from build123d import *

# Parameters (mm, degrees)
BOSS_EXTRUDE1_DEPTH     = 30
SKETCH3_R               = 1.4
CUT_EXTRUDE1_DEPTH      = 5
MIRROR2_COPY_1_SKETCH_R = 1.4
MIRROR2_COPY_1_DEPTH    = 5


with BuildPart() as part:
    # Sketch2 → Boss-Extrude1 (new body)
    with BuildSketch(Plane(origin=(0, 0, 0), x_dir=(1, 0, 0), z_dir=(0, 1, 0))):
        with BuildLine():
            ThreePointArc((6.25, 13.635890143), (0, 15), (-6.25, 13.635890143))
            ThreePointArc((-6.25, 13.635890143), (-7.727178029, 9.658712115), (-3.75, 8.181534086))
            ThreePointArc((-3.75, 8.181534086), (0, 9), (3.75, 8.181534086))
            ThreePointArc((3.75, 8.181534086), (7.727178029, 9.658712115), (6.25, 13.635890143))
        make_face()
    extrude(amount=BOSS_EXTRUDE1_DEPTH)

    # Sketch3 → Cut-Extrude1 (cut)
    with BuildSketch(Plane(origin=(0, 30, 0), x_dir=(1, 0, 0), z_dir=(0, 1, 0))):
        with Locations(Location((5, 10.908712115, 0), (0, 0, 270))):
            Circle(SKETCH3_R)
    cut_extrude1 = extrude(amount=-CUT_EXTRUDE1_DEPTH, mode=Mode.SUBTRACT)

    # Mirror1: Cut-Extrude1 across plane
    add(cut_extrude1.mirror(Plane(origin=(0, 0, 0), x_dir=(0, 0, 1), z_dir=(1, 0, 0))), mode=Mode.SUBTRACT)

    # Mirror2: Cut-Extrude1 across plane
    add(cut_extrude1.mirror(Plane.ZX.offset(15)), mode=Mode.SUBTRACT)

    # Mirror2 copy 1 sketch → Mirror2 copy 1 (cut)
    with BuildSketch(Plane(origin=(0, 0, 0), x_dir=(-1, 0, 0), z_dir=(0, -1, 0))):
        with Locations(Location((5, 10.908712115, 0), (0, 0, 270))):
            Circle(MIRROR2_COPY_1_SKETCH_R)
    extrude(amount=-MIRROR2_COPY_1_DEPTH, mode=Mode.SUBTRACT)


solid = part.part
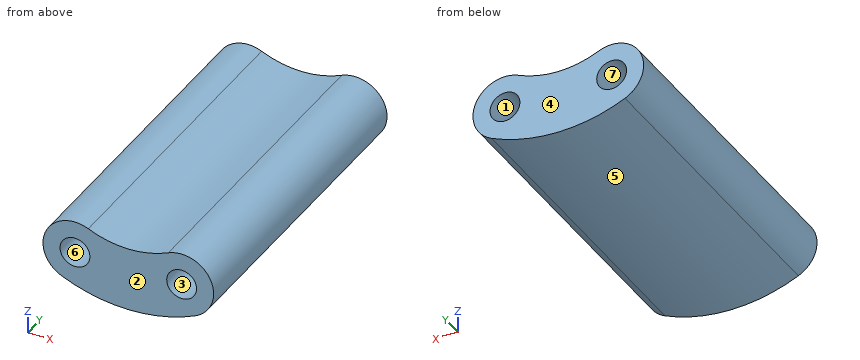
Design review of the part built by this model. Coordinates are the model's own, in mm. Face numbers are marked on the shaded views. A direction names the side the tool comes from. Give positions to 0.01 mm unless a question says otherwise; leave off trailing zeros. Loops run counter-clockwise (first coordinate to the right, second up) from the corner with the lowest first, then second, coordinate; pieces in that order, holes last. Notation, with made-up numbers: (9, 84.5) - (31, 84.5) arc R20 ccw to (31, 102.5) - close; hole circle Ø9 at (-24, 18). An arc over 180 degrees is marked (long way). Use CSV: the item, a comma, the result in double quotes. Start each with the question number.
1. Insertion check: P1, Ø6, axis at x = 5, y = 18.5, coming from the -Z side; P2, Ø1.4, axis at x = 5, z = -11.5, coming from the +Y side; P3, Ø3, axis at x = -4, y = 21.5, coming from the -Z side. Each pin has a flat end and moves straight along its axis. Give the tip position at first contact, or say it passes through.
2. Add section A-A (z = -8.5). State the section outline as (x, y) points.
3. Add section D-D (z = -11). State the section outline as (x, y) points, plus the area to 3 significant figures.
4. Wall thickness on L1, parallel to X at y = 2.25, z = -10.75; L2, parallel to X at y = 13.5, z = -11; L3, parallel to Y at x = -5.25, z = -9.75: over which ranges is each line inside the solid? List them lowest first.
5. Draft analysis for pull direction X (two halves, no side actions). For the marked faces 4, 5, 6 and 7, state which applies: released by +X, released by -X, zero draft, split by the parting line, or undercut.
6. Add section C-C (x = -5). State the section outline as (y, z) points, plus the area to 3 significant figures.
7. Machinability: for the marked faces 1, 2 and 3, which of the approach directions +Z, -Z, +X, -X, +Y, -Y give a long, thin tool a straight path to every point of the face, cutting with its end or side? Answer none if there is none.
8. Add section B-B (y = 14.75). State the section outline as (x, z) points.
Results found:
1,P1,"stops at z = -14.87"
1,P2,"stops at y = 25"
1,P3,"stops at z = -14.79"
2,outline,"(-6.79, 0) - (-2.96, 0) - (-2.96, 30) - (-6.79, 30) - close; (2.96, 0) - (6.79, 0) - (6.79, 30) - (2.96, 30) - close"
3,outline,"(-8, 0) - (-6.4, 0) - (-6.4, 5) - (-3.6, 5) - (-3.6, 0) - (3.6, 0) - (3.6, 5) - (6.4, 5) - (6.4, 0) - (8, 0) - (8, 30) - (6.4, 30) - (6.4, 25) - (3.6, 25) - (3.6, 30) - (-3.6, 30) - (-3.6, 25) - (-6.4, 25) - (-6.4, 30) - (-8, 30) - close"
3,area,"424 mm²"
4,L1,"x = -8 to -6.39, -3.61 to 3.61, 6.39 to 8"
4,L2,"x = -8 to 8"
4,L3,"y = 5 to 25"
5,face 4,"zero draft"
5,face 5,"split by the parting line"
5,face 6,"undercut"
5,face 7,"undercut"
6,outline,"(0, -14.14) - (30, -14.14) - (30, -12.31) - (25, -12.31) - (25, -9.51) - (30, -9.51) - (30, -7.91) - (0, -7.91) - (0, -9.51) - (5, -9.51) - (5, -12.31) - (0, -12.31) - close"
6,area,"159 mm²"
7,face 1,"+Y"
7,face 2,"+Z, -Z, +X, -X, -Y"
7,face 3,"-Y"
8,outline,"(-6.25, -13.64) arc R15 ccw to (6.25, -13.64) arc R3 ccw to (3.75, -8.18) arc R9 cw to (-3.75, -8.18) arc R3 ccw to start"
